from build123d import *

# Parameters (mm, degrees)
SKETCH3_R           = 2.6035
BOSS_EXTRUDE1_DEPTH = 9.398
CUT_EXTRUDE1_START  = -3.3528
SKETCH4_R           = 14.605
SKETCH4_R_2         = 2.6035
SKETCH4_R_3         = 13.0175
CUT_EXTRUDE1_DEPTH  = 3.3528
SKETCH5_R           = 13.843
BOSS_EXTRUDE2_DEPTH = 7.747
SKETCH6_R           = 8.4455
BOSS_EXTRUDE3_DEPTH = 1.905
SKETCH7_R           = 8.509
BOSS_EXTRUDE4_DEPTH = 34.798
CUT_EXTRUDE2_DEPTH  = 47.503968347
FILLET1_R           = 3.175
CHAMFER1_SIZE       = 1.905
SKETCH9_R           = 6.6675
BOSS_EXTRUDE5_DEPTH = 0.762
CUT_EXTRUDE3_DEPTH  = 11.43
CHAMFER2_SIZE       = 3.175
FILLET2_R           = 1.27


with BuildPart() as part:
    # Sketch3 → Boss-Extrude1 (new body)
    with BuildSketch(Plane(origin=(0, 0, 0), x_dir=(1, 0, 0), z_dir=(0, 1, 0))):
        with BuildLine():
            ThreePointArc((18.41992125, -4.85890946), (26.2509, 0), (18.41992125, 4.85890946))
            ThreePointArc((18.41992125, 4.85890946), (0, 19.05), (-18.41992125, 4.85890946))
            ThreePointArc((-18.41992125, 4.85890946), (-26.2509, 0), (-18.41992125, -4.85890946))
            ThreePointArc((-18.41992125, -4.85890946), (0, -19.05), (18.41992125, -4.85890946))
        make_face()
        with Locations(Location((-20.828, 0, 0), (0, 0, 270))):
            Circle(SKETCH3_R, mode=Mode.SUBTRACT)
        with Locations(Location((20.828, 0, 0), (0, 0, 270))):
            Circle(SKETCH3_R, mode=Mode.SUBTRACT)
    extrude(amount=BOSS_EXTRUDE1_DEPTH)

    # Sketch4 → Cut-Extrude1 (cut)
    # profile 1 of 2: a face of its own
    with BuildSketch(Plane(origin=(0, 9.398, 0), x_dir=(1, 0, 0), z_dir=(0, 1, 0)).offset(CUT_EXTRUDE1_START)):
        with BuildLine():
            ThreePointArc((-18.41992125, 4.85890946), (-26.2509, 0), (-18.41992125, -4.85890946))
            ThreePointArc((-18.41992125, -4.85890946), (0, -19.05), (18.41992125, -4.85890946))
            ThreePointArc((18.41992125, -4.85890946), (26.2509, 0), (18.41992125, 4.85890946))
            ThreePointArc((18.41992125, 4.85890946), (0, 19.05), (-18.41992125, 4.85890946))
        make_face()
        with Locations(Location((0, 0, 0), (0, 0, 270))):
            Circle(SKETCH4_R, mode=Mode.SUBTRACT)
        with Locations(Location((20.828, 0, 0), (0, 0, 270))):
            Circle(SKETCH4_R_2, mode=Mode.SUBTRACT)
        with Locations(Location((-20.828, 0, 0), (0, 0, 270))):
            Circle(SKETCH4_R_2, mode=Mode.SUBTRACT)
    # profile 2 of 2: a face of its own
    with BuildSketch(Plane(origin=(0, 9.398, 0), x_dir=(1, 0, 0), z_dir=(0, 1, 0)).offset(CUT_EXTRUDE1_START)):
        with Locations(Location((0, 0, 0), (0, 0, 270))):
            Circle(SKETCH4_R_3)
    extrude(amount=CUT_EXTRUDE1_DEPTH, mode=Mode.SUBTRACT)

    # Sketch5 → Boss-Extrude2 (add)
    with BuildSketch(Plane.XZ):
        with Locations(Location((0, 0, 0), (0, 0, 270))):
            Circle(SKETCH5_R)
    extrude(amount=BOSS_EXTRUDE2_DEPTH)

    # Sketch6 → Boss-Extrude3 (add)
    with BuildSketch(Plane.XZ.offset(7.747)):
        with Locations(Location((0, 0, 0), (0, 0, 90))):
            Circle(SKETCH6_R)
    extrude(amount=BOSS_EXTRUDE3_DEPTH)

    # Sketch7 → Boss-Extrude4 (add)
    with BuildSketch(Plane.XY):
        with Locations(Location((0, -1.651, 0), (0, 0, 168.811944249))):
            Circle(SKETCH7_R)
    extrude(amount=BOSS_EXTRUDE4_DEPTH)

    # Sketch8 → Cut-Extrude2 (cut, through all)
    with BuildSketch(Plane(origin=(0, 6.0452, 0), x_dir=(1, 0, 0), z_dir=(0, 1, 0))):
        with BuildLine():
            Line((-3.629268047, 0), (-3.629268047, -12.501348715))
            ThreePointArc((-3.629268047, -12.501348715), (0, -13.0175), (3.629268047, -12.501348715))
            Line((3.629268047, -12.501348715), (3.629268047, 0))
            Line((3.629268047, 0), (-3.629268047, 0))
        make_face()
        with BuildLine():
            ThreePointArc((-3.629268047, -18.70109391), (0, -19.05), (3.629268047, -18.70109391))
            Line((3.629268047, -18.70109391), (3.629268047, -14.146887942))
            ThreePointArc((3.629268047, -14.146887942), (0, -14.605), (-3.629268047, -14.146887942))
            Line((-3.629268047, -14.146887942), (-3.629268047, -18.70109391))
        make_face()
    extrude(amount=CUT_EXTRUDE2_DEPTH, mode=Mode.SUBTRACT)

    # Fillet1
    fillet1_edges = [part.edges().sort_by_distance(p)[0] for p in [
        (-18.41992125, 3.0226, 4.85890946),
        (-18.41992125, 3.0226, -4.85890946),
        (18.41992125, 3.0226, -4.85890946),
        (18.41992125, 3.0226, 4.85890946),
    ]]
    fillet(fillet1_edges, radius=FILLET1_R)

    # Chamfer1
    chamfer1_edges = [part.edges().sort_by_distance(p)[0] for p in [
        (0, -9.652, -8.4455),
    ]]
    chamfer(chamfer1_edges, length=CHAMFER1_SIZE - 0.0001)  # a hair under: the kernel refuses the full size

    # Sketch9 → Boss-Extrude5 (add)
    with BuildSketch(Plane(origin=(0, 6.0452, 0), x_dir=(1, 0, 0), z_dir=(0, 1, 0))):
        with Locations(Location((0, 0, 0), (0, 0, 90))):
            Circle(SKETCH9_R)
    extrude(amount=BOSS_EXTRUDE5_DEPTH)

    # Sketch10 → Cut-Extrude3 (cut)
    with BuildSketch(Plane(origin=(0, 6.8072, 0), x_dir=(1, 0, 0), z_dir=(0, 1, 0))):
        with BuildLine():
            Line((-2.171634675, 4.380777681), (4.380777681, -2.171634675))
            ThreePointArc((4.380777681, -2.171634675), (-3.457398607, -3.457398607), (-2.171634675, 4.380777681))
        make_face()
    extrude(amount=-CUT_EXTRUDE3_DEPTH, mode=Mode.SUBTRACT)

    # Chamfer2
    chamfer2_edges = [part.edges().sort_by_distance(p)[0] for p in [
        (1.104571503, 6.8072, -1.104571503),
    ]]
    chamfer(chamfer2_edges, length=CHAMFER2_SIZE)

    # Fillet2
    fillet2_edges = [part.edges().sort_by_distance(p)[0] for p in [
        (0, -7.747, -13.843),
    ]]
    fillet(fillet2_edges, radius=FILLET2_R)


solid = part.part
Input: part model. Units: mm. Frame: model coordinates. A direction names the side the tool comes from. Give positions to 0.01 mm unless a question says otherwise; leave off trailing zeros. Order: outer loops, then holes, each group sorted by start corner. A loop starts at its lowest first (then second) coordinate and runs counter-clockwise, first axis right, second up. Notation, with made-up numbers: M 38.5,-17 L 91.5,-17 A20 cw 91.5,1 Z; hole C 6,15.25 d11. An arc over 180 degrees is marked long. Answer as a JSON object with one key per item and string values.
1. Reachability of faces 1 (the cylindrical face through (-18.247, 2.98, -0.339)), 2 (the flat face through (-1, -4.623, 1)), 3 (the cylindrical face through (-0.55, -10.142, 21.022)) from +Z, -Z, +X, -X, +Y, -Y: full face, straight path, thin tool, end or side. Return the list, or none.
Result sheet:
{"face 1": "+Y, -Y", "face 2": "+Y", "face 3": "+Z"}
2. Cut plane C-C, the plane y = -3. Output: boundary loops of the cut face in (x, z), and give its area (3 significant figures).
Result sheet:
{"outline": "M -8.4,11 A13.84 ccw long 8.4,11 L 8.4,34.8 L -8.4,34.8 Z; hole M -2.17,-4.38 L 4.38,2.17 A4.89 ccw long Z", "area": "917 mm²"}
3. Cut plane D-D, the plane y = 1.5. State how many separate pieces and enclosed holes the cut face has, and give its area (3 significant figures).
Result sheet:
{"separate pieces": "1", "enclosed holes": "3", "area": "1,440 mm²"}
4. Ray query, line 1 (Z direction, x = 0, y = 7.2) (1 decimal); line 2 (Y direction, x = 3, z = -15.5); line 3 (X direction, y = 7.25, z = -2). Return the intervals inside material, ascending. Write a range as [from, to].
Result sheet:
{"line 1": "[-14.6, -13], [13, 14.6]", "line 2": "[0, 6.05]", "line 3": "[-14.47, -12.86], [12.86, 14.47]"}
5. First-contact query: P1, Ø1, axis at x = -10.5, y = 2, coming from the -Z side; P2, Ø4, axis at x = -11.5, z = 5, coming from the -Y side; P3, Ø8.5, axis at x = -20.828, z = 0, coming from the +Y side. Flat tips, straight axial feed; report the tip coordinate or a pass-through.
Result sheet:
{"P1": "z = -16.21", "P2": "y = -7.75", "P3": "y = 6.05"}
6. Cut plane B-B, the plane y = 7.75. Output: boundary loops of the cut face in (x, z) (1 decimal).
Result sheet:
{"outline": "C 0,0 d29.2; hole C 0,0 d26"}
7. Pull-direction query (X, two-part tool) for faces 4 (the flat face through (0, -2, 34.798)), 5 (the cylindrical face through (13.466, 2.98, 13.475)), 6 (the cylindrical face through (-3.315, 1.172, 3.594)); classes: +X half, -X half, draft (parallel to the pull), parting line (faces both ways), or undercut.
Result sheet:
{"face 4": "draft", "face 5": "+X half", "face 6": "undercut"}
